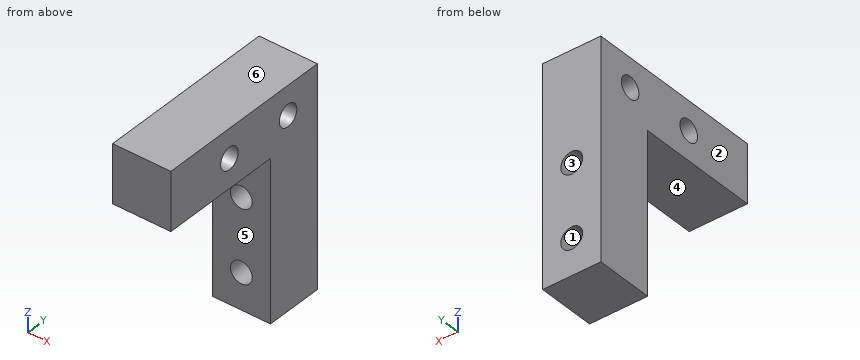
from build123d import *

# Parameters (mm, degrees)
BOSS_EXTRUDE1_DEPTH = 8
SKETCH2_R           = 3
CUT_EXTRUDE1_DEPTH  = 58.861904566
SKETCH3_R           = 3
CUT_EXTRUDE2_DEPTH  = 68.082039325


with BuildPart() as part:
    # Sketch1 → Boss-Extrude1 (new, symmetric)
    with BuildSketch(Plane(origin=(0, 0, 0), x_dir=(0, 0, -1), z_dir=(1, 0, 0))):
        Polygon((0, 0), (0, -34), (-16, -34), (-16, 16), (44, 16), (44, 0), align=None)
    extrude(amount=BOSS_EXTRUDE1_DEPTH, both=True)

    # Sketch2 → Cut-Extrude1 (cut, through all)
    with BuildSketch(Plane(origin=(8, 0, 0), x_dir=(0, 0, -1), z_dir=(1, 0, 0))):
        with Locations((-8, 6)):
            Circle(SKETCH2_R)
        with Locations((-8, -14)):
            Circle(SKETCH2_R)
    extrude(amount=-CUT_EXTRUDE1_DEPTH, mode=Mode.SUBTRACT)

    # Sketch3 → Cut-Extrude2 (cut, through all)
    with BuildSketch(Plane(origin=(0, 16, 0), x_dir=(1, 0, 0), z_dir=(0, 1, 0))):
        with Locations(Location((0, 34, 0), (0, 0, 270))):
            Circle(SKETCH3_R)
        with Locations(Location((0, 14, 0), (0, 0, 270))):
            Circle(SKETCH3_R)
    extrude(amount=-CUT_EXTRUDE2_DEPTH, mode=Mode.SUBTRACT)


solid = part.part
The listing builds one solid part. Answer for the finished solid, in the listing's coordinates (mm). Face numbers are marked on the shaded views. A direction names the side the tool comes from. Give positions to 0.01 mm unless a question says otherwise; leave off trailing zeros. Order: outer loops, then holes, each group sorted by start corner. A loop starts at its lowest first (then second) coordinate and runs counter-clockwise, first axis right, second up. Notation, with made-up numbers: (26, -33.5) -> (63, -33.5) arc R25 ccw to (63, 4.5) -> close; hole circle Ø10 at (30.25, 80). An arc over 180 degrees is marked (long way). Put each result on its own line as item: value.
Item 1: For a pull along Z with two mould halves and no side action, classify the marked faces 1, 2, 3 and 4 as released by +Z, released by -Z, zero draft, split by the parting line, or undercut.
Established:
face 1: undercut
face 2: zero draft
face 3: undercut
face 4: released by -Z
Item 2: Given P1, Ø8, axis at y = -1.5, z = -34, coming from the -X side; P2, Ø4, axis at x = 1, y = -24, coming from the -Z side; P3, Ø3.5, axis at y = 6, z = 8, coming from the -X side; P4, Ø7, axis at x = 0, z = -34, coming from the -Y side, each flat-ended and moving along its own axis, determine where each tip first touches the part or whether it passes through.
Established:
P1: stops at x = -8
P2: stops at z = 0
P3: passes through
P4: stops at y = 0
Item 3: A cutting plane is placed at D-D on y = -14. Give the vertices of the cut face in (x, z).
Established:
outline: (-8, 0) -> (8, 0) -> (8, 5) -> (-8, 5) -> close; (-8, 11) -> (8, 11) -> (8, 16) -> (-8, 16) -> close
Item 4: A cutting plane is placed at A-A on y = 6. Give the vertices of the cut face in (x, z).
Established:
outline: (-8, -44) -> (8, -44) -> (8, 5) -> (-8, 5) -> close; (-8, 11) -> (8, 11) -> (8, 16) -> (-8, 16) -> close; hole circle Ø6 at (0, -34); hole circle Ø6 at (0, -14)
Item 5: For the marked faces 5 and 6, determine the directions among +Z, -Z, +X, -X, +Y, -Y from which every point of the face is accessible in a straight line to the end or side of a thin tool.
Established:
face 5: -Z, +X, -X, -Y
face 6: +Z, +X, -X, +Y, -Y
Item 6: Straight lines are drawn through the part: line 1 (Y direction, x = -3, z = 8); line 2 (X direction, y = 4, z = -34); line 3 (Z direction, x = 1.5, y = 14). For each, find the intervals that lie inside material, in ascending order.
Established:
line 1: y = -34 to -17, -11 to 3, 9 to 16
line 2: x = -8 to -3, 3 to 8
line 3: z = -44 to -36.6, -31.4 to -16.6, -11.4 to 16
Item 7: A cutting plane is placed at C-C on z = 8. Give the vertices of the cut face in (x, y).
Established:
outline: (-8, -34) -> (8, -34) -> (8, -17) -> (-8, -17) -> close; (-8, -11) -> (8, -11) -> (8, 3) -> (-8, 3) -> close; (-8, 9) -> (8, 9) -> (8, 16) -> (-8, 16) -> close
Item 8: A cutting plane is placed at B-B on x = 0. Give the vertices of the cut face in (y, z).
Established:
outline: (-34, 0) -> (0, 0) -> (0, -11) -> (16, -11) -> (16, 16) -> (-34, 16) -> close; (0, -44) -> (16, -44) -> (16, -37) -> (0, -37) -> close; (0, -31) -> (16, -31) -> (16, -17) -> (0, -17) -> close; hole circle Ø6 at (-14, 8); hole circle Ø6 at (6, 8)
